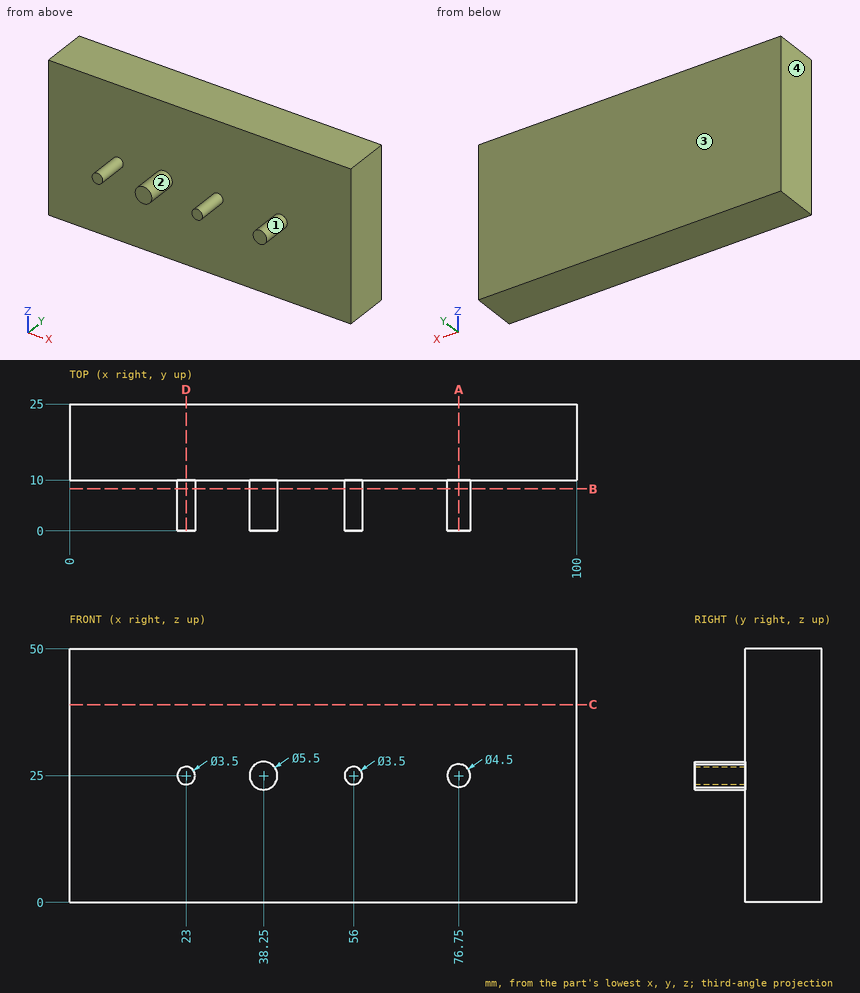
Source: three-view drawing plus pictorial views. Frame: mm from the lowest corner of the part. Round coordinates to 2 decimals unless told otherwise and drop trailing zeros. Order: outer loops, then holes, each group sorted by start corner. A loop starts at its lowest first (then second) coordinate and runs counter-clockwise, first axis right, second up. Notation, with made-up numbers: (9, 29) - (64, 29) arc R10 ccw to (64, 43) - close; hole circle Ø5 at (13, 3). An arc over 180 degrees is marked (long way). Write each question's results on one line, items separated by ' | '.
Item 1: Section B-B, the plane y = 8.25. Return the cut outline in (x, z).
Completed:
outline: circle Ø3.5 at (23, 25); circle Ø5.5 at (38.25, 25); circle Ø3.5 at (56, 25); circle Ø4.5 at (76.75, 25)
Item 2: First-contact query: pin 1 Ø5 at (y, z) = (6.5, 25.5) entering from +X; pin 2 Ø3 at (y, z) = (3.5, 28) entering from -X; pin 3 Ø3 at (x, z) = (48, 37.5) entering from -Y. Flat tips, straight axial feed; report the tip coordinate or a pass-through.
Completed:
pin 1: x = 79 | pin 2: x = 22.1 | pin 3: y = 10
Item 3: Section D-D, the plane x = 23. Return the cut outline in (y, z).
Completed:
outline: (0, 23.25) - (10, 23.25) - (10, 0) - (25, 0) - (25, 50) - (10, 50) - (10, 26.75) - (0, 26.75) - close
Item 4: Section A-A, the plane x = 76.75. Return the cut outline in (y, z).
Completed:
outline: (0, 22.75) - (10, 22.75) - (10, 0) - (25, 0) - (25, 50) - (10, 50) - (10, 27.25) - (0, 27.25) - close
Item 5: Section C-C, the plane z = 39. Return the cut outline in (x, y), and give its area (3 significant figures).
Completed:
outline: (0, 10) - (100, 10) - (100, 25) - (0, 25) - close | area: 1,500 mm^2
Item 6: Mould query, pull axis X, two halves, no side actions, for the marked faces 1, 2, 3 and 4. Classes: pulls with the +X half, pulls with the -X half, needs draft (parallel to the pull), parting line crosses it, or undercut.
Completed:
face 1: undercut | face 2: undercut | face 3: needs draft | face 4: pulls with the -X half
Item 7: Material intervals for line 1 along Y through (x, z) = (83, 34), sorted ascending. Write a range as [from, to].
Completed:
line 1: [10, 25]
